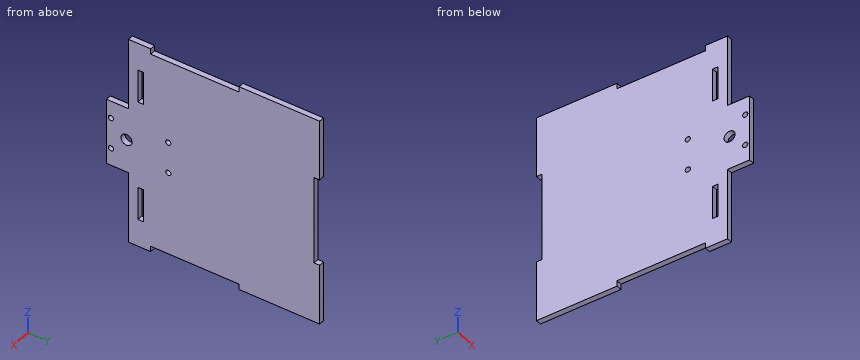
Autodesk Inventor part; units mm, degrees
ref_plane "YZ Plane" through (0, 0, 0) normal (1, 0, 0) x (0, 1, 0)
ref_plane "XZ Plane" through (0, 0, 0) normal (0, 1, 0) x (-1, 0, 0)
ref_plane "XY Plane" through (0, 0, 0) normal (0, 0, 1) x (1, 0, 0)
sketch "Sketch1" plane through (0, 0, 0) normal (1, 0, 0) x (0, 1, 0)
  line L0 (0, 0) -> (97.4344, 0)
  line L1 (97.4344, 0) -> (97.4344, -114.3)
  line L2 (97.4344, -114.3) -> (0, -114.3)
  line L3 (0, -114.3) -> (0, 0)
  dimension "d0" = 114.3
  dimension "d1" = 97.4344
extrude "Extrusion1" add sketch "Sketch1" along normal blind 3.175
sketch "Sketch2" plane through (3.175, 0, 0) normal (1, 0, 0) x (0, 0, -1)
  circle A0 centre (48.1457, 35.5346) radius 1.4986
  circle A1 centre (66.1543, 35.5346) radius 1.4986
  circle A2 centre (66.1543, 2.54) radius 1.4986
  circle A3 centre (48.1457, 2.54) radius 1.4986
  line L0 (114.3, 0) -> (114.3, 97.4344)
  line L1 (0, 0) -> (114.3, 0)
  line L2 (0, 0) -> (0, 97.4344)
  dimension "d4" = 18.0086
  dimension "d5" = 2.9972
  dimension "d6" = 2.9972
  dimension "d7" = 2.9972
  dimension "d8" = 2.9972
  dimension "d11" = 18.0086
  dimension "d12" = 2.54
  dimension "d28" = 2.54
  dimension "d29" = 32.9946
  dimension "d30" = 32.9946
  dimension "d65" = 48.1457
extrude "Extrusion2" cut sketch "Sketch2" against normal blind 3.175
sketch "Sketch3" plane through (3.175, 0, 0) normal (1, 0, 0) x (0, 0, -1)
  circle A0 centre (57.15, 11.5316) radius 3.175
  line L0 (114.3, 0) -> (114.3, 97.4344)
  circle A1 centre (66.1543, 2.54) radius 1.4986
  point P0 (0, 0)
  dimension "d15" = 6.35
  dimension "d16" = 57.15
  dimension "d17" = 8.9916
extrude "Extrusion3" cut sketch "Sketch3" against normal blind 3.175 contours A0
sketch "Sketch4" plane through (3.175, 0, 0) normal (1, 0, 0) x (0, 0, -1)
  line L0 (0, 97.4344) -> (0, 0)
  line L1 (0, 0) -> (114.3, 0)
  line L2 (114.3, 0) -> (114.3, 97.4344)
  line L3 (31.75, 18.0594) -> (12.7, 18.0594)
  line L4 (12.7, 18.0594) -> (12.7, 21.2344)
  line L5 (12.7, 21.2344) -> (31.75, 21.2344)
  line L6 (31.75, 21.2344) -> (31.75, 18.0594)
  circle A0 centre (57.15, 11.5316) radius 3.175
  line L7 (57.15, 11.5316) -> (57.15, 79.1299) construction
  line L8 (82.55, 18.0594) -> (101.6, 18.0594)
  line L9 (101.6, 18.0594) -> (101.6, 21.2344)
  line L10 (101.6, 21.2344) -> (82.55, 21.2344)
  line L11 (82.55, 21.2344) -> (82.55, 18.0594)
  point P0 (12.7, 0)
  point P1 (31.75, 0)
  point P2 (101.6, 0)
  dimension "d31" = 3.175
  dimension "d33" = 19.05
  dimension "d34" = 12.7
  dimension "d43" = 18.0594
extrude "Extrusion5" cut sketch "Sketch4" against normal blind 3.175 contours L3 L4 L5 L6 | L11 L10 L9 L8
sketch "Sketch5" plane through (3.175, 0, 0) normal (1, 0, 0) x (0, 0, -1)
  line L0 (0, 0) -> (38.1, 0)
  line L1 (38.1, 0) -> (38.1, 12.7)
  line L2 (38.1, 12.7) -> (0, 12.7)
  line L3 (0, 12.7) -> (0, 0)
  line L4 (114.3, 0) -> (0, 0)
  line L5 (114.3, 0) -> (76.2, 0)
  line L6 (76.2, 0) -> (76.2, 12.7)
  line L7 (76.2, 12.7) -> (114.3, 12.7)
  line L8 (114.3, 12.7) -> (114.3, 0)
  dimension "d37" = 38.1
  dimension "d38" = 12.7
  dimension "d39" = 38.1
  dimension "d42" = 12.7
extrude "Extrusion6" cut sketch "Sketch5" against normal blind 3.175
sketch "Sketch6" plane through (3.175, 0, 0) normal (1, 0, 0) x (0, 0, -1)
  line L0 (0, 97.4344) -> (0, 12.7)
  line L1 (0, 69.85) -> (3.175, 69.85)
  line L2 (3.175, 69.85) -> (3.175, 50.8)
  line L3 (3.175, 50.8) -> (0, 50.8)
  line L4 (0, 50.8) -> (0, 69.85)
  line L5 (0, 12.7) -> (38.1, 12.7)
  line L6 (38.1, 0) -> (76.2, 0)
  line L7 (57.15, 0) -> (57.15, 76.8026) construction
  line L8 (114.3, 97.4344) -> (114.3, 12.7)
  line L9 (114.3, 69.85) -> (111.125, 69.85)
  line L10 (111.125, 69.85) -> (111.125, 50.8)
  line L11 (111.125, 50.8) -> (114.3, 50.8)
  line L12 (114.3, 50.8) -> (114.3, 69.85)
  point P0 (0, 0)
  dimension "d44" = 38.1
  dimension "d45" = 19.05
  dimension "d46" = 3.175
extrude "Extrusion7" cut sketch "Sketch6" against normal blind 3.175
sketch "Sketch7" plane through (3.175, 0, 0) normal (1, 0, 0) x (0, 0, -1)
  line L0 (0, 101.4731) -> (-3.175, 101.4731)
  line L1 (-3.175, 101.4731) -> (-3.175, 12.7)
  line L2 (-3.175, 12.7) -> (0, 12.7)
  line L3 (0, 12.7) -> (0, 101.4731)
  line L4 (114.3, 50.8) -> (114.3, 12.7)
  line L5 (114.3, 12.7) -> (117.475, 12.7)
  line L6 (117.475, 12.7) -> (117.475, 101.4731)
  line L7 (117.475, 101.4731) -> (114.3, 101.4731)
  line L8 (114.3, 101.4731) -> (114.3, 12.7)
  line L9 (0, 97.4344) -> (0, 69.85)
  line L10 (0, 69.85) -> (3.3446, 69.85)
  line L11 (3.3446, 69.85) -> (3.3446, 50.8)
  line L12 (3.3446, 50.8) -> (0, 50.8)
  line L13 (0, 50.8) -> (0, 69.85)
  line L14 (111.125, 69.85) -> (111.125, 50.8)
  line L15 (111.125, 69.85) -> (114.3, 69.85)
  line L16 (114.3, 69.85) -> (114.3, 50.8)
  line L17 (114.3, 50.8) -> (111.125, 50.8)
  line L18 (111.125, 50.8) -> (111.125, 69.85)
  line L19 (0, 97.4344) -> (-3.175, 97.4344)
  line L20 (0, 97.4344) -> (114.3, 97.4344)
  line L21 (114.3, 97.4344) -> (117.475, 97.4344)
  point P0 (0, 0)
  dimension "d49" = 3.175
  dimension "d50" = 3.175
  dimension "d51" = 0
extrude "Extrusion8" add sketch "Sketch7" against normal blind 3.175
sketch "Sketch8" plane through (3.175, 0, 0) normal (1, 0, 0) x (0, 0, -1)
  line L0 (-3.175, 101.4731) -> (-3.175, 12.7)
  line L1 (-3.175, 76.2) -> (0, 76.2)
  line L2 (0, 76.2) -> (0, 25.4)
  line L3 (0, 25.4) -> (-3.175, 25.4)
  line L4 (-3.175, 25.4) -> (-3.175, 76.2)
  line L5 (117.475, 101.4731) -> (117.475, 12.7)
  line L6 (117.475, 76.2) -> (114.3, 76.2)
  line L7 (114.3, 76.2) -> (114.3, 25.4)
  line L8 (114.3, 25.4) -> (117.475, 25.4)
  line L9 (117.475, 25.4) -> (117.475, 76.2)
  line L10 (-3.175, 12.7) -> (38.1, 12.7)
  point P0 (0, 0)
  dimension "d54" = 3.175
  dimension "d55" = 3.175
  dimension "d56" = 50.8
  dimension "d57" = 50.8
  dimension "d58" = 12.7
extrude "Extrusion9" cut sketch "Sketch8" against normal blind 3.175
sketch "Sketch9" plane through (3.175, 0, 0) normal (1, 0, 0) x (0, 0, -1)
  line L0 (-3.175, 76.2) -> (-3.175, 101.4731)
  line L1 (-3.175, 97.0871) -> (127.7131, 97.0871)
  line L2 (127.7131, 97.0871) -> (127.7131, 110.1997)
  line L3 (127.7131, 110.1997) -> (-3.175, 110.1997)
  line L4 (-3.175, 110.1997) -> (-3.175, 97.0871)
  point P0 (0, 0)
extrude "Extrusion10" cut sketch "Sketch9" against normal blind 3.175
sketch "Sketch10" plane through (0, 0, 0) normal (-1, 0, 0) x (0, 0, 1)
  line L0 (-117.475, 97.0871) -> (-117.475, 76.2)
  line L1 (-117.475, 97.0871) -> (3.175, 97.0871)
  line L2 (3.175, 97.0871) -> (3.175, 122.4871)
  line L3 (3.175, 122.4871) -> (-117.475, 122.4871)
  line L4 (-117.475, 122.4871) -> (-117.475, 97.0871)
  line L5 (3.175, 76.2) -> (3.175, 97.0871)
  point P0 (0, 0)
  dimension "d66" = 0
  dimension "d67" = 25.4
extrude "Extrusion11" add sketch "Sketch10" against normal blind 3.175
sketch "Sketch11" plane through (3.175, 0, 0) normal (1, 0, 0) x (0, 0, -1)
  line L0 (117.475, 122.4871) -> (-3.175, 122.4871)
  line L1 (31.75, 122.4871) -> (82.55, 122.4871)
  line L2 (82.55, 122.4871) -> (82.55, 119.3121)
  line L3 (82.55, 119.3121) -> (31.75, 119.3121)
  line L4 (31.75, 119.3121) -> (31.75, 122.4871)
  line L5 (-3.175, 122.4871) -> (-3.175, 76.2)
  point P0 (0, 0)
  dimension "d70" = 50.8
  dimension "d71" = 3.175
  dimension "d72" = 34.925
extrude "Extrusion12" cut sketch "Sketch11" against normal blind 3.175
properties part number "side"
Geometry check sheet. Reference: the model listing, model coordinates, mm. Give positions to 0.01 mm unless a question says otherwise; leave off trailing zeros. Write each loop counter-clockwise with the first axis right and the second up, starting at its lowest first coordinate (ties: lowest second). Pieces come first, ordered by that corner, then holes. Notation, with made-up numbers: M 88,82 L 103,82 A16 ccw 103,112 Z; hole C 21,-39.5 d6. An arc over 180 degrees is marked long. Answer as CSV lines item,"result". Start each with the question number.
Q1. Section check A-A, the plane y = 2.54. Record the cut outline in (x, z) (3 decimals), then the cut area to 3 significant figures.
Q2. Section check C-C, the plane x = 0.9. Give the number of separate pieces and of enclosed holes in the cut face, then the cut area to 3 significant figures.
Q3. Go/stop test with flat-tipped pins: pin 1 (2.5 mm diameter, centred on y = 2.54, z = -66.15, fed in from -X); pin 2 (1 mm diameter, centred on x = 2, z = -115.5, fed in from -Y); pin 3 (1.6 mm diameter, centred on x = 1, y = 58.5, fed in from -Z); pin 4 (1.5 mm diameter, centred on y = 99.5, z = -25, fed in from -X). Record where each tip stops, or that it passes through.
Q4. Section check D-D, the plane z = -74. Record the cut outline in (x, y) (3 decimals).
Q5. Material ranges on L1, parallel to Y at x = 2.4, z = -87; L2, parallel to Y at x = 2.3, z = -57.15; L3, parallel to Z at x = 2.4, y = 56.5, recorded low to high.
Q6. Section check B-B, the plane z = -57.15. Record the cut outline in (x, y) (3 decimals), then the cut area to 3 significant figures.
Geometry says:
1,outline,"M 0,-76.2 L 3.175,-76.2 L 3.175,-67.653 L 0,-67.653 Z; M 0,-64.656 L 3.175,-64.656 L 3.175,-49.644 L 0,-49.644 Z; M 0,-46.647 L 3.175,-46.647 L 3.175,-38.1 L 0,-38.1 Z"
1,area,"102 mm^2"
2,separate pieces,"1"
2,enclosed holes,"7"
2,area,"13,100 mm^2"
3,pin 1,"through"
3,pin 2,"y = 12.7"
3,pin 3,"z = -114.3"
3,pin 4,"x = 0"
4,outline,"M 0,0 L 3.175,0 L 3.175,119.312 L 0,119.312 Z"
5,L1,"12.7 to 18.06, 21.23 to 122.49"
5,L2,"0 to 8.36, 14.71 to 119.31"
5,L3,"-114.3 to 0"
6,outline,"M 0,0 L 3.175,0 L 3.175,8.357 L 0,8.357 Z; M 0,14.707 L 3.175,14.707 L 3.175,119.312 L 0,119.312 Z"
6,area,"359 mm^2"
